Geometry check sheet. Reference: the model listing, model coordinates, mm. Face numbers are marked on the shaded views. A direction names the side the tool comes from. Round coordinates to 2 decimals unless told otherwise and drop trailing zeros. Loops run counter-clockwise (first coordinate to the right, second up) from the corner with the lowest first, then second, coordinate; pieces in that order, holes last. Notation, with made-up numbers: M 84.5,87 L 116.5,87 A32 cw 116.5,125 Z; hole C 3,7 d7. An arc over 180 degrees is marked long. Write item = value, one per line.
from build123d import *

# Parameters (mm, degrees)
ESQUISSE1_W                  = 42.5
ESQUISSE1_H                  = 42.5
BOSS_EXTRU_1_DEPTH           = 5
ESQUISSE2_R                  = 1.325
ENL_V_MAT_EXTRU_1_DEPTH      = 31.465144017
ENL_V_MAT_EXTRU_2_DEPTH      = 31.465144017
ESQUISSE4_W                  = 42.5
ESQUISSE4_H                  = 19.1
BOSS_EXTRU_2_DEPTH           = 5
ESQUISSE5_W                  = 42.5
ESQUISSE5_H                  = 8
BOSS_EXTRU_3_DEPTH           = 16
ESQUISSE7_R                  = 2.6
ENL_V_MAT_EXTRU_3_DEPTH      = 49.578132941
CONG_2_R                     = 1
CHANFREIN1_SIZE              = 4
CONG_2_OF_SYM_TRIE3_R        = 1
CHANFREIN1_OF_SYM_TRIE3_SIZE = 4
ESQUISSE11_R                 = 4.325
ENL_V_MAT_EXTRU_4_DEPTH      = 5
ENL_V_MAT_EXTRU_5_DEPTH      = 5
ENL_V_MAT_EXTRU_6_DEPTH      = 50.958332638
ENL_V_MAT_EXTRU_7_DEPTH      = 50.958332638
ENL_V_MAT_EXTRU_8_DEPTH      = 5
SYM_TRIE5_COPY_1_SKETCH_R    = 4.325
SYM_TRIE5_COPY_1_DEPTH       = 5


with BuildPart() as part:
    # Esquisse1 → Boss.-Extru.1 (new body)
    with BuildSketch(Plane(origin=(0, 0, 0), x_dir=(1, 0, 0), z_dir=(0, 1, 0))):
        Rectangle(ESQUISSE1_W, ESQUISSE1_H)
    extrude(amount=BOSS_EXTRU_1_DEPTH)

    # Esquisse2 → Enlèv. mat.-Extru.1 (cut, through all)
    with BuildSketch(Plane(origin=(0, 5, 0), x_dir=(1, 0, 0), z_dir=(0, 1, 0))):
        with Locations(Location((-15.5, 15.5, 0), (0, 0, 270))):
            Circle(ESQUISSE2_R)
        with Locations(Location((15.5, 15.5, 0), (0, 0, 270))):
            Circle(ESQUISSE2_R)
    enl_v_mat_extru_1 = extrude(amount=-ENL_V_MAT_EXTRU_1_DEPTH, mode=Mode.SUBTRACT)

    # Symétrie1: Enlèv. mat.-Extru.1 across plane
    add(enl_v_mat_extru_1.mirror(Plane.XY), mode=Mode.SUBTRACT)

    # Esquisse3 → Enlèv. mat.-Extru.2 (cut, through all)
    with BuildSketch(Plane(origin=(0, 5, 0), x_dir=(1, 0, 0), z_dir=(0, 1, 0))):
        with BuildLine():
            Line((2.424108484, 11.752603884), (0, 12.252603884))
            Line((0, 12.252603884), (-2.424108484, 11.752603884))
            ThreePointArc((-2.424108484, 11.752603884), (0, -12), (2.424108484, 11.752603884))
        make_face()
    extrude(amount=-ENL_V_MAT_EXTRU_2_DEPTH, mode=Mode.SUBTRACT)

    # Esquisse4 → Boss.-Extru.2 (add)
    with BuildSketch(Plane(origin=(21.25, 0, 0), x_dir=(0, 0, -1), z_dir=(1, 0, 0))):
        with Locations((0, -4.55)):
            Rectangle(ESQUISSE4_W, ESQUISSE4_H)
    boss_extru_2 = extrude(amount=BOSS_EXTRU_2_DEPTH)

    # Esquisse5 → Boss.-Extru.3 (add)
    with BuildSketch(Plane(origin=(26.25, 0, 0), x_dir=(0, 0, -1), z_dir=(1, 0, 0))):
        with Locations((0, -10.1)):
            Rectangle(ESQUISSE5_W, ESQUISSE5_H)
    boss_extru_3 = extrude(amount=BOSS_EXTRU_3_DEPTH)

    # Esquisse7 → Enlèv. mat.-Extru.3 (cut, through all)
    with BuildSketch(Plane(origin=(0, -6.1, 0), x_dir=(1, 0, 0), z_dir=(0, 1, 0))):
        with Locations(Location((35.75, 15, 0), (0, 0, 270))):
            Circle(ESQUISSE7_R)
        with Locations(Location((35.75, -15, 0), (0, 0, 270))):
            Circle(ESQUISSE7_R)
    enl_v_mat_extru_3 = extrude(amount=-ENL_V_MAT_EXTRU_3_DEPTH, mode=Mode.SUBTRACT)

    # Congé2
    cong_2_edges = [part.edges().sort_by_distance(p)[0] for p in [
        (26.25, 5, 0),
        (42.25, -6.1, 0),
    ]]
    fillet(cong_2_edges, radius=CONG_2_R)

    # Chanfrein1
    chanfrein1_edges = [part.edges().sort_by_distance(p)[0] for p in [
        (26.25, -6.1, 0),
    ]]
    chamfer(chanfrein1_edges, length=CHANFREIN1_SIZE)

    # Symétrie3: Boss.-Extru.2, Boss.-Extru.3, Enlèv. mat.-Extru.3 across plane
    add(boss_extru_2.mirror(Plane(origin=(0, 0, 0), x_dir=(0, 0, 1), z_dir=(1, 0, 0))))
    add(boss_extru_3.mirror(Plane(origin=(0, 0, 0), x_dir=(0, 0, 1), z_dir=(1, 0, 0))))
    add(enl_v_mat_extru_3.mirror(Plane(origin=(0, 0, 0), x_dir=(0, 0, 1), z_dir=(1, 0, 0))), mode=Mode.SUBTRACT)

    # Congé2 of Symétrie3
    cong_2_of_sym_trie3_edges = [part.edges().sort_by_distance(p)[0] for p in [
        (-26.25, 5, 0),
        (-42.25, -6.1, 0),
    ]]
    fillet(cong_2_of_sym_trie3_edges, radius=CONG_2_OF_SYM_TRIE3_R)

    # Chanfrein1 of Symétrie3
    chanfrein1_of_sym_trie3_edges = [part.edges().sort_by_distance(p)[0] for p in [
        (-26.25, -6.1, 0),
    ]]
    chamfer(chanfrein1_of_sym_trie3_edges, length=CHANFREIN1_OF_SYM_TRIE3_SIZE)

    # Esquisse11 → Enlèv. mat.-Extru.4 (cut)
    with BuildSketch(Plane(origin=(0, -6.1, 0), x_dir=(1, 0, 0), z_dir=(0, 1, 0))):
        with Locations(Location((35.75, 15, 0), (0, 0, 270))):
            Circle(ESQUISSE11_R)
    enl_v_mat_extru_4 = extrude(amount=-ENL_V_MAT_EXTRU_4_DEPTH, mode=Mode.SUBTRACT)

    # Symétrie4: Enlèv. mat.-Extru.4 across plane
    add(enl_v_mat_extru_4.mirror(Plane.XY), mode=Mode.SUBTRACT)

    # Esquisse12 → Enlèv. mat.-Extru.5 (cut)
    with BuildSketch(Plane(origin=(0, -6.1, 0), x_dir=(1, 0, 0), z_dir=(0, 1, 0))):
        Polygon((37.178674107, 19.082219408), (34.321325893, 19.082219408), (35.75, 19.582219408), align=None)
    enl_v_mat_extru_5 = extrude(amount=-ENL_V_MAT_EXTRU_5_DEPTH, mode=Mode.SUBTRACT)

    # Esquisse13 → Enlèv. mat.-Extru.6 (cut, through all)
    with BuildSketch(Plane(origin=(0, -11.1, 0), x_dir=(1, 0, 0), z_dir=(0, 1, 0))):
        Polygon((34.663263699, 17.361991577), (36.836736301, 17.361991577), (35.75, 17.861991577), align=None)
    enl_v_mat_extru_6 = extrude(amount=-ENL_V_MAT_EXTRU_6_DEPTH, mode=Mode.SUBTRACT)

    # Esquisse14 → Enlèv. mat.-Extru.7 (cut, through all)
    with BuildSketch(Plane(origin=(0, -11.1, 0), x_dir=(1, 0, 0), z_dir=(0, 1, 0))):
        Polygon((36.836736301, -12.638008423), (35.75, -12.138008423), (34.663263699, -12.638008423), align=None)
    enl_v_mat_extru_7 = extrude(amount=-ENL_V_MAT_EXTRU_7_DEPTH, mode=Mode.SUBTRACT)

    # Esquisse15 → Enlèv. mat.-Extru.8 (cut)
    with BuildSketch(Plane(origin=(0, -6.1, 0), x_dir=(1, 0, 0), z_dir=(0, 1, 0))):
        Polygon((34.321325893, -10.917780592), (37.178674107, -10.917780592), (35.75, -10.417780592), align=None)
    enl_v_mat_extru_8 = extrude(amount=-ENL_V_MAT_EXTRU_8_DEPTH, mode=Mode.SUBTRACT)

    # Symétrie5: Enlèv. mat.-Extru.4, Enlèv. mat.-Extru.5, Enlèv. mat.-Extru.6, Enlèv. mat.-Extru.7, Enlèv. mat.-Extru.8 across plane
    add(enl_v_mat_extru_4.mirror(Plane(origin=(0, 0, 0), x_dir=(0, 0, 1), z_dir=(1, 0, 0))), mode=Mode.SUBTRACT)
    add(enl_v_mat_extru_5.mirror(Plane(origin=(0, 0, 0), x_dir=(0, 0, 1), z_dir=(1, 0, 0))), mode=Mode.SUBTRACT)
    add(enl_v_mat_extru_6.mirror(Plane(origin=(0, 0, 0), x_dir=(0, 0, 1), z_dir=(1, 0, 0))), mode=Mode.SUBTRACT)
    add(enl_v_mat_extru_7.mirror(Plane(origin=(0, 0, 0), x_dir=(0, 0, 1), z_dir=(1, 0, 0))), mode=Mode.SUBTRACT)
    add(enl_v_mat_extru_8.mirror(Plane(origin=(0, 0, 0), x_dir=(0, 0, 1), z_dir=(1, 0, 0))), mode=Mode.SUBTRACT)

    # Symétrie5 copy 1 sketch → Symétrie5 copy 1 (cut)
    with BuildSketch(Plane(origin=(0, -6.1, 0), x_dir=(-1, 0, 0), z_dir=(0, 1, 0))):
        with Locations(Location((35.75, 15, 0), (0, 0, 270))):
            Circle(SYM_TRIE5_COPY_1_SKETCH_R)
    extrude(amount=-SYM_TRIE5_COPY_1_DEPTH, mode=Mode.SUBTRACT)


solid = part.part
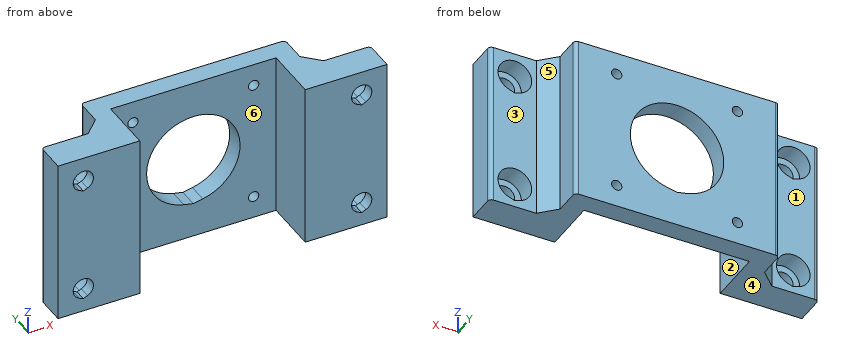
(1) Sectioned sample at C-C on y = 2.5. Record the cut outline in (x, z) (3 decimals), then the cut area to 3 significant figures.
Result set:
outline = M -26.25,-21.25 L 26.25,-21.25 L 26.25,21.25 L -26.25,21.25 Z; hole C -15.5,-15.5 d2.65; hole C -15.5,15.5 d2.65; hole M -2.424,-11.753 L 0,-12.253 L 2.424,-11.753 A12 ccw long Z; hole C 15.5,-15.5 d2.65; hole C 15.5,15.5 d2.65
area = 1,760 mm2
(2) Release check for a two-part mould opening along X. For the marked faces 4, 5 and 6 record: released by +X, released by -X, zero draft, split by the parting line, or undercut.
Result set:
face_4 = zero draft
face_5 = released by +X
face_6 = undercut
(3) Sectioned sample at B-B on x = -15.5. Record the cut outline in (y, z) (3 decimals), then the cut area to 3 significant figures.
Result set:
outline = M 0,-21.25 L 5,-21.25 L 5,-16.825 L 0,-16.825 Z; M 0,-14.175 L 5,-14.175 L 5,14.175 L 0,14.175 Z; M 0,16.825 L 5,16.825 L 5,21.25 L 0,21.25 Z
area = 186 mm2
(4) Tool access check on the marked faces 1, 2 and 3. Record the directions out of +Z, -Z, +X, -X, +Y, -Y that give a thin tool (end or side, any length) a straight path to the whole face; none if there is none.
Result set:
face_1 = +Z, -Z, -X, +Y
face_2 = +Z, -Z, -Y
face_3 = +Z, -Z, +X, +Y
(5) Material ranges on line 1 along X through (y, z) = (-7.25, 15) (3 decimals); line 2 along Z through (x, y) = (35.75, -11.75); line 3 along X through (y, z) = (-12.25, 15), recorded low to high. Write a range as from..to.
Result set:
line_1 = -42.25..-40.075, -31.425..-21.25, 21.25..31.425, 40.075..42.25
line_2 = -21.25..-17.86, -12.4..12.14, 17.6..21.25
line_3 = -42.25..-38.35, -33.15..-21.25, 21.25..33.15, 38.35..42.25
(6) Sectioned sample at D-D on z = -7. Record the cut outline in (x, y), then the cut area to 3 significant figures.
Result set:
outline = M -42.25,-14.1 L -21.25,-14.1 L -21.25,0 L -9.75,0 L -9.75,5 L -25.25,5 A1 ccw -26.25,4 L -26.25,-2.1 L -30.25,-6.1 L -41.25,-6.1 A1 ccw -42.25,-7.1 Z; M 9.75,0 L 21.25,0 L 21.25,-14.1 L 42.25,-14.1 L 42.25,-7.1 A1 ccw 41.25,-6.1 L 30.25,-6.1 L 26.25,-2.1 L 26.25,4 A1 ccw 25.25,5 L 9.75,5 Z
area = 577 mm2
(7) Depth check by flat-ended pin: pin 1 Ø4 at (x, z) = (-15.5, 15.5) entering from -Y; pin 2 Ø3 at (y, z) = (-1, -16) entering from -X; pin 3 Ø12 at (x, z) = (-37.5, 6.5) entering from +Y. Enter the tip coordinate at first touch or a pass-through.
Result set:
pin_1 = 0
pin_2 = -26.65
pin_3 = -6.1
(8) Sectioned sample at A-A on y = -8. Record the cut outline in (x, z) (3 decimals).
Result set:
outline = M -42.25,-21.25 L -21.25,-21.25 L -21.25,21.25 L -42.25,21.25 Z; M 21.25,-21.25 L 42.25,-21.25 L 42.25,21.25 L 21.25,21.25 Z; hole M -37.179,-19.082 L -35.75,-19.582 L -34.321,-19.082 A4.325 ccw long Z; hole M -37.179,10.918 L -35.75,10.418 L -34.321,10.918 A4.325 ccw long Z; hole M 34.321,-19.082 L 35.75,-19.582 L 37.179,-19.082 A4.325 ccw long Z; hole M 34.321,10.918 L 35.75,10.418 L 37.179,10.918 A4.325 ccw long Z
